```python
from build123d import *

# Parameters (mm, degrees)
F0_W     = 12.75
F0_H     = 6
F1_DEPTH = 6
F2_R     = 1.389063
F3_DEPTH = 12.751
F4_R     = 1.339063
F5_DEPTH = 6.35
F6_R     = 0.508


with BuildPart() as f1:
    # F0 (on Top) → F1 (new body, symmetric)
    with BuildSketch(Plane.XY):
        Rectangle(F0_W, F0_H)
    extrude(amount=F1_DEPTH, both=True)

    # F2 (on face) → F3 (cut, through all)
    with BuildSketch(Plane.YZ.offset(6.375)):
        Circle(F2_R)
    extrude(amount=-F3_DEPTH, mode=Mode.SUBTRACT)

    # F4 (on face) → F5 (cut)
    with BuildSketch(Plane.XY.offset(6)):
        with Locations((-3.175, 0)):
            Circle(F4_R)
        with Locations((3.175, 0)):
            Circle(F4_R)
    extrude(amount=-F5_DEPTH, mode=Mode.SUBTRACT)

    # F6
    f6_edges = [f1.edges().sort_by_distance(p)[0] for p in [
        (0, 3, -6),
        (6.375, 3, 0),
        (6.375, 0, -6),
        (6.375, -3, 0),
        (0, -3, -6),
        (-6.375, 0, -6),
        (-6.375, 3, 0),
        (-6.375, -3, 0),
    ]]
    fillet(f6_edges, radius=F6_R)


solid = f1.part
```
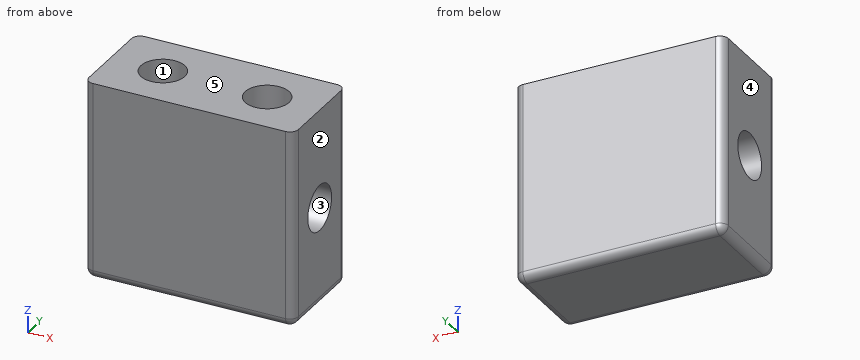
The listing builds one solid part. Answer for the finished solid, in the listing's coordinates (mm). Face numbers are marked on the shaded views. A direction names the side the tool comes from. Give positions to 0.01 mm unless a question says otherwise; leave off trailing zeros. Order: outer loops, then holes, each group sorted by start corner. A loop starts at its lowest first (then second) coordinate and runs counter-clockwise, first axis right, second up. Notation, with made-up numbers: (43, 56.25) -> (74, 56.25) arc R25 ccw to (74, 68.25) -> close; hole circle Ø7 at (-4, 11). An arc over 180 degrees is marked (long way). Answer as a JSON object with one key per item and string values. Group by question number.
Item 1: The part is cut by section C-C on y = 0. Write down the section's boundary in (x, z) (3 decimals).
Item 2: Consider L1, parallel to X at y = 0, z = 3.4 (3 decimals); L2, parallel to Z at x = -0.75, y = -0.1; L3, parallel to Z at x = 6.25, y = 0.55. Determine where each line is inside the solid, lowest interval first. Write a range as from..to.
Item 3: A flat-ended cylindrical pin translates along its axis: pin 1 (1.6 mm diameter, centred on x = -3.175, y = 0, fed in from +Z). Find the tip coordinate at first contact, or state that the pin passes through.
Item 4: The part is cut by section A-A on z = 0. Write down the section's boundary in (x, y) (3 decimals).
Item 5: A tool of negligible diameter and unlimited length cuts with its end or side. For the marked faces 1 and 2, from which of +Z, -Z, +X, -X, +Y, -Y can it reach the whole face along a straight path? Write none if from no direction.
Item 6: Determine the mould class of the marked faces 3, 4 and 5 for opening direction Z: pulls with the +Z half, pulls with the -Z half, needs draft (parallel to the pull), parting line crosses it, or undercut.
Item 7: The part is cut by section D-D on z = 3.25. Write down the section's boundary in (x, y) (3 decimals), and give its area (3 significant figures).
Item 8: The part is cut by section B-B on x = 1. Write down the section's boundary in (y, z), and give its area (3 significant figures).
Result set:
{
 "1": {"outline": "(-6.375, -5.492) arc R0.508 ccw to (-5.867, -6) -> (5.867, -6) arc R0.508 ccw to (6.375, -5.492) -> (6.375, -1.389) -> (-6.375, -1.389) -> close; (-6.375, 1.389) -> (-4.514, 1.389) -> (-4.514, 6) -> (-6.375, 6) -> close; (-1.836, 1.389) -> (1.836, 1.389) -> (1.836, 6) -> (-1.836, 6) -> close; (4.514, 1.389) -> (6.375, 1.389) -> (6.375, 6) -> (4.514, 6) -> close"},
 "2": {"L1": "-6.375..-4.514, -1.836..1.836, 4.514..6.375", "L2": "-6..-1.39, 1.39..6", "L3": "-5.83..-1.28, 1.28..6"},
 "3": {"pin 1": "z = -1.14"},
 "4": {"outline": "(-6.375, -2.492) arc R0.508 ccw to (-5.867, -3) -> (5.867, -3) arc R0.508 ccw to (6.375, -2.492) -> (6.375, -1.389) -> (-6.375, -1.389) -> close; (-6.375, 1.389) -> (6.375, 1.389) -> (6.375, 2.492) arc R0.508 ccw to (5.867, 3) -> (-5.867, 3) arc R0.508 ccw to (-6.375, 2.492) -> close"},
 "5": {"face 1": "+Z", "face 2": "+Z, -Z, +X, +Y, -Y"},
 "6": {"face 3": "undercut", "face 4": "needs draft", "face 5": "pulls with the +Z half"},
 "7": {"outline": "(-6.375, -2.492) arc R0.508 ccw to (-5.867, -3) -> (5.867, -3) arc R0.508 ccw to (6.375, -2.492) -> (6.375, 2.492) arc R0.508 ccw to (5.867, 3) -> (-5.867, 3) arc R0.508 ccw to (-6.375, 2.492) -> close; hole circle Ø2.678 at (-3.175, 0); hole circle Ø2.678 at (3.175, 0)", "area": "65.0 mm²"},
 "8": {"outline": "(-3, -5.49) arc R0.51 ccw to (-2.49, -6) -> (2.49, -6) arc R0.51 ccw to (3, -5.49) -> (3, 6) -> (-3, 6) -> close; hole circle Ø2.78 at (0, 0)", "area": "65.8 mm²"}
}
